Autodesk Inventor part; units mm, degrees
ref_plane "YZ Plane" through (0, 0, 0) normal (1, 0, 0) x (0, 1, 0)
ref_plane "XZ Plane" through (0, 0, 0) normal (0, 1, 0) x (-1, 0, 0)
ref_plane "XY Plane" through (0, 0, 0) normal (0, 0, 1) x (1, 0, 0)
sketch "Sketch1" plane through (0, 0, 0) normal (0, 0, 1) x (1, 0, 0)
  circle A0 centre (-14.977, 17.3579) radius 26.4414
  point P0 (0, 0)
  dimension "d0" = 52.8828
extrude "Extrusion1" add sketch "Sketch1" along normal blind 18.7198
chamfer "Chamfer1" distance 1.5875 angle 45 1 edges at (-41.4184, 17.3579, 18.7198)
sketch "Sketch2" plane through (-14.977, 17.3579, 18.7198) normal (0, 0, 1) x (1, 0, 0)
  circle A0 centre (0, 0) radius 24.8539
  circle A1 centre (0, 0) radius 26.4414
  line L0 (-21.1455, -15.875) -> (21.1455, -15.875)
  line L1 (-21.1455, 15.875) -> (21.1455, 15.875)
  arc A2 (21.1455, 15.875) -> (-21.1455, 15.875) centre (0, 0) ccw
  arc A3 (-21.1455, -15.875) -> (21.1455, -15.875) centre (0, 0) ccw
  point P0 (14.977, -17.3579)
  dimension "d6" = 31.75
  dimension "d7" = 15.875
extrude "Extrusion2" cut sketch "Sketch2" against normal blind 8.128 contours L1 A0 | A0 L1 A1 | L0 A1 A0 | A0 L0
sketch "Sketch3" plane through (0, 0, 18.7198) normal (0, 0, 1) x (1, 0, 0)
  arc A0 (-34.1003, 33.2329) -> (-34.1003, 1.4829) centre (-14.977, 17.3579) ccw
  circle A1 centre (-14.977, 17.3579) radius 5.3975
  point P0 (0, 0)
  dimension "d10" = 10.795
extrude "Extrusion3" cut sketch "Sketch3" against normal through all
thread "Thread1"
properties part number "Auumulator Cap 1764"
Could you check a few things on this model? Use its own coordinates, in mm. A direction names the side the tool comes from. Coordinates: 2 decimals unless noted, no trailing zeros. Write each loop counter-clockwise with the first axis right and the second up, starting at its lowest first coordinate (ties: lowest second). Pieces come first, ordered by that corner, then holes. Notation, with made-up numbers: M 41.5,5.25 L 96.5,5.25 A29 ccw 96.5,29.25 Z; hole C 62,50.5 d5. An arc over 180 degrees is marked long. Answer as CSV lines item,"result". Start each with the question number.
1) For P1, Ø9, axis at x = -10, z = 15.5, coming from the +Y side; P2, Ø11.5, axis at x = -18, y = 37, coming from the +Z side; P3, Ø3, axis at x = -1, z = 8.5, coming from the +Y side; P4, Ø1, axis at y = 4, z = 5.5, coming from the +X side, each with a flat end and sliding along its axis, tell me the tip position at first contact or that it passes through.
2) I want a section at B-B, the plane z = 13. Please give me the cut outline in (x, y) (1 decimal), and give its area (3 significant figures).
3) I want a section at A-A, the plane x = -12. Please give me the cut outline in (y, z), and give its area (3 significant figures).
4) Please list where these lines run through material, in increasing order: line 1 (X direction, y = 18, z = 2); line 2 (Z direction, x = -0.5, y = -3.5); line 3 (Y direction, x = 5.5, z = 12.25). Write a range as from..to.
5) For faces 5 (the flat face through (-15, 37, 10.592)), 6 (the flat face through (-15, -3, 10.592)), 7 (the flat face through (-9, 18, 0)), which set-ups out of +Z, -Z, +X, -X, +Y, -Y let a thin tool reach every point of the face, with its end or its side?
6) I want a section at D-D, the plane y = -1.5. Please give me the cut outline in (x, z), and give its area (3 significant figures).
7) We'd pull the mould along Y, two halves only. Please class faces 1 (the flat face through (-15, 1.483, 15)), 2 (the cylindrical face through (10.243, 9.416, 6.543)), 3 (the flat face through (-15, 33.233, 15)), 4 (the cylindrical face through (-20.37, 17.6, 9.49)): +Y half, -Y half, draft (parallel to the pull), parting line (faces both ways), or undercut.
8) I want a section at C-C, the plane x = -29.5. Please give me the cut outline in (y, z), and give its area (3 significant figures).
Data:
1,P1,"stops at y = 33.23"
1,P2,"stops at z = 18.72"
1,P3,"stops at y = 40.67"
1,P4,"stops at x = 8.13"
2,outline,"M -36.1,1.5 L 6.2,1.5 A26.4 ccw 6.2,33.2 L -36.1,33.2 A26.4 ccw Z; hole C -15,17.4 d10.8"
2,area,"1,480 mm^2"
3,outline,"M -8.92,0 L 12.86,0 L 12.86,18.72 L 1.48,18.72 L 1.48,10.59 L -8.92,10.59 Z; M 21.86,0 L 43.63,0 L 43.63,10.59 L 33.23,10.59 L 33.23,18.72 L 21.86,18.72 Z"
3,area,"646 mm^2"
4,line 1,"x = -41.41..-20.34, -9.62..11.46"
4,line 2,"z = 0..10.59"
4,line 3,"y = 1.48..33.23"
5,face 5,"+Z, +X, -X, +Y"
5,face 6,"+Z, +X, -X, -Y"
5,face 7,"-Z, +X, -X, +Y, -Y"
6,outline,"M -33.51,0 L 3.56,0 L 3.56,10.59 L -33.51,10.59 Z"
6,area,"393 mm^2"
7,face 1,"-Y half"
7,face 2,"parting line"
7,face 3,"+Y half"
7,face 4,"undercut"
8,outline,"M -4.74,0 L 39.45,0 L 39.45,10.59 L 33.23,10.59 L 33.23,18.72 L 1.48,18.72 L 1.48,10.59 L -4.74,10.59 Z"
8,area,"726 mm^2"
